Job drawing, mm, ordinate dimensions from the low corner. One solid piece. A direction names the side the tool comes from. Coordinates: 2 decimals unless noted, no trailing zeros. Write each loop counter-clockwise with the first axis right and the second up, starting at its lowest first coordinate (ties: lowest second). Pieces come first, ordered by that corner, then holes. Notation, with made-up numbers: (79.5, 6) -> (98.5, 6) arc R19 cw to (98.5, 23) -> close; hole circle Ø8 at (-31, -11.75). An arc over 180 degrees is marked (long way). Answer as a JSON object with one key per item and string values. Group by question number.
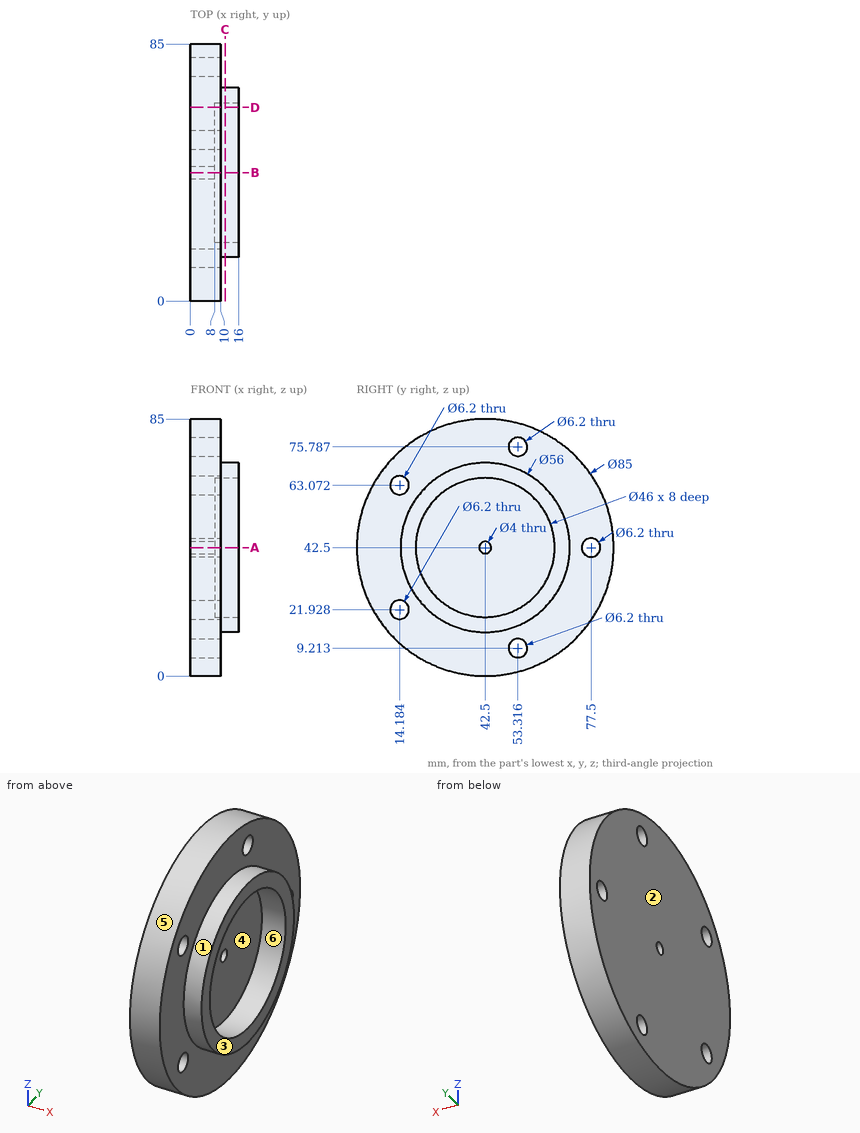
(1) Cut at B-B on y = 42.5. List the corners of the cut face in (x, z).
(2) Pull direction Y, two halves, no side cores. Call the marked faces 3, 4, 5 and 6: released by +Y, released by -Y, zero draft, split by the parting line, or undercut.
(3) Cut at A-A on z = 42.5. List the corners of the cut face in (x, y), plus the area to 3 significant figures.
(4) Wall check: probe 1 along Z at (x, y) = (5, 50.5) (1 decimal); probe 2 along X at (y, z) = (49.5, 25); probe 3 along X at (y, z) = (29.5, 17). Give the ranges that are in metal, low to high.
(5) 3-axis set-ups, long thin cutter, end or side, ignore diameter. For the marked faces 1 and 2: which of +Z, -Z, +X, -X, +Y, -Y reach the whole face in a straight line?
(6) Cut at C-C on x = 11.5. List the corners of the cut face in (y, z).
(7) Pin check, flat tips, straight feed: pin 1 (4 mm diameter, centred on y = 27.5, z = 26, fed in from +X); pin 2 (1 mm diameter, centred on x = 12.5, z = 62, fed in from -Y); pin 3 (14 mm diameter, centred on y = 36.5, z = 44.5, fed in from +X); pin 4 (10 mm diameter, centred on y = 53.32, z = 75.79, fed in from +X). Stop position of each tip, or through.
(8) Cut at D-D on y = 64. List the corners of the cut face in (x, z), plus the area to 3 significant figures.
Results found:
{
 "1": {"outline": "(0, 0) -> (10, 0) -> (10, 14.5) -> (16, 14.5) -> (16, 19.5) -> (8, 19.5) -> (8, 40.5) -> (0, 40.5) -> close; (0, 44.5) -> (8, 44.5) -> (8, 65.5) -> (16, 65.5) -> (16, 70.5) -> (10, 70.5) -> (10, 85) -> (0, 85) -> close"},
 "2": {"face 3": "zero draft", "face 4": "undercut", "face 5": "split by the parting line", "face 6": "undercut"},
 "3": {"outline": "(0, 0) -> (10, 0) -> (10, 14.5) -> (16, 14.5) -> (16, 19.5) -> (8, 19.5) -> (8, 40.5) -> (0, 40.5) -> close; (0, 44.5) -> (8, 44.5) -> (8, 65.5) -> (16, 65.5) -> (16, 70.5) -> (10, 70.5) -> (10, 74.4) -> (0, 74.4) -> close; (0, 80.6) -> (10, 80.6) -> (10, 85) -> (0, 85) -> close", "area": "724 mm²"},
 "4": {"probe 1": "z = 0.8 to 7.9, 10.5 to 74.5, 77.1 to 84.2", "probe 2": "x = 0 to 8", "probe 3": "x = 0 to 10"},
 "5": {"face 1": "+X", "face 2": "+Z, -Z, -X, +Y, -Y"},
 "6": {"outline": "circle Ø56 at (42.5, 42.5); hole circle Ø46 at (42.5, 42.5)"},
 "7": {"pin 1": "stops at x = 16", "pin 2": "stops at y = 21.93", "pin 3": "stops at x = 8", "pin 4": "stops at x = 10"},
 "8": {"outline": "(0, 5.84) -> (10, 5.84) -> (10, 24.56) -> (16, 24.56) -> (16, 34.33) -> (8, 34.33) -> (8, 50.67) -> (16, 50.67) -> (16, 60.44) -> (10, 60.44) -> (10, 79.16) -> (0, 79.16) -> close", "area": "818 mm²"}
}
